Geometry: final body of the model. Coordinates: model frame, mm. Give positions to 0.01 mm unless a question says otherwise; leave off trailing zeros. Write each loop counter-clockwise with the first axis right and the second up, starting at its lowest first coordinate (ties: lowest second). Pieces come first, ordered by that corner, then holes. Notation, with made-up numbers: M -8,57.25 L 11,57.25 A28 ccw 11,93.25 Z; hole C 51,-1 d4. An arc over 180 degrees is marked long. Use a Markdown table: item, result. Add a question column.
1) Line query: line 1 (X direction, y = 36.5, z = 0.1); line 2 (Y direction, x = 25.5, z = 2.05); line 3 (Y direction, x = -25, z = 1.6). Output: solid intervals per line, ascending.
2) Pin query (flat end, axial travel): pin 1 (0.8 mm diameter, centred on x = 27.5, z = 1, fed in from +Y); pin 2 (0.8 mm diameter, centred on y = 20, z = 1.5, fed in from -X); pin 3 (1.5 mm diameter, centred on y = 12, z = 0.5, fed in from +X). Return the tip coordinate at first contact, or that it passes through.
3) Section B-B on y = 14. Return the cut outline in (x, z).
4) Section A-A on y = -15.5. Return the cut outline in (x, z), then the cut area to 3 significant figures.
```python
from build123d import *

# Parameters (mm, degrees)
F0_W        = 9.75
F0_H        = 13.75
F1_DEPTH    = 2.5
F0_W_2      = 2.5
F0_H_2      = 8
F2_DEPTH    = 1.75
F3_R        = 2
F4_R        = 5
F5_T1_DEPTH = 23.4006350946


# Not quite as in the source:
# - a fillet or chamfer that OpenCascade refuses, or shapes differently, is made with other operations: its cross-section is extruded or revolved along the edge and cut away or added


with BuildPart() as f1:
    # F0 (on Top) → F1 (new body)
    with BuildSketch(Plane.XY):
        Polygon((25.0968417823, 39.3397479696), (-25.4031582177, 39.3397479696), (-25.4031582177, 30.0897479696), (-25.4031582177, 22.0897479696), (-25.4031582177, -4.6602520304), (-25.4031582177, -12.6602520304), (-25.4031582177, -21.9102520304), (25.0968417823, -21.9102520304), (25.0968417823, 1.8397479696), (25.0968417823, 15.5897479696), align=None)
        with Locations((29.9718417823, 8.7147479696)):
            Rectangle(F0_W, F0_H)
    extrude(amount=F1_DEPTH)

    # F0 (on Top) → F2 (join)
    with BuildSketch(Plane.XY):
        with Locations((-26.6531582177, 26.0897479696)):
            Rectangle(F0_W_2, F0_H_2)
        with Locations((-26.6531582177, -8.6602520304)):
            Rectangle(F0_W_2, F0_H_2)
    extrude(amount=F2_DEPTH)

    # F3
    f3_edges = [f1.edges().sort_by_distance(p)[0] for p in [
        (-25.403158, 39.339748, 1.25),
        (-25.403158, -21.910252, 1.25),
        (25.096842, -21.910252, 1.25),
        (25.096842, 39.339748, 1.25),
    ]]
    fillet(f3_edges, radius=F3_R)

    # F4
    f4_edges = [f1.edges().sort_by_distance(p)[0] for p in [
        (34.846842, 1.839748, 1.25),
        (34.846842, 15.589748, 1.25),
    ]]
    fillet(f4_edges, radius=F4_R)

    # F5: fillet of radius 5 on 4 edges, made by hand

    # F5_s2 → F5_t1 (cut)
    with BuildSketch(Plane.XY.offset(-10.8253175473)):
        with BuildLine():
            ThreePointArc((-25.4031582177, 30.0897479696), (-27.2332852366, 28.2596209506), (-27.9031582177, 25.7596209506))
            Line((-27.9031582177, 25.7596209506), (-27.9031582177, 30.0897479696))
            Line((-27.9031582177, 30.0897479696), (-25.4031582177, 30.0897479696))
        make_face()
        with BuildLine():
            ThreePointArc((-27.9031582177, 26.4198749885), (-27.2332852366, 23.9198749885), (-25.4031582177, 22.0897479696))
            Line((-25.4031582177, 22.0897479696), (-27.9031582177, 22.0897479696))
            Line((-27.9031582177, 22.0897479696), (-27.9031582177, 26.4198749885))
        make_face()
        with BuildLine():
            ThreePointArc((-25.4031582177, -4.6602520304), (-27.2332852366, -6.4903790494), (-27.9031582177, -8.9903790494))
            Line((-27.9031582177, -8.9903790494), (-27.9031582177, -4.6602520304))
            Line((-27.9031582177, -4.6602520304), (-25.4031582177, -4.6602520304))
        make_face()
        with BuildLine():
            ThreePointArc((-25.4031582177, -12.6602520304), (-27.2332852366, -10.8301250115), (-27.9031582177, -8.3301250115))
            Line((-27.9031582177, -8.3301250115), (-27.9031582177, -12.6602520304))
            Line((-27.9031582177, -12.6602520304), (-25.4031582177, -12.6602520304))
        make_face()
    extrude(amount=F5_T1_DEPTH, mode=Mode.SUBTRACT)


solid = f1.part
```
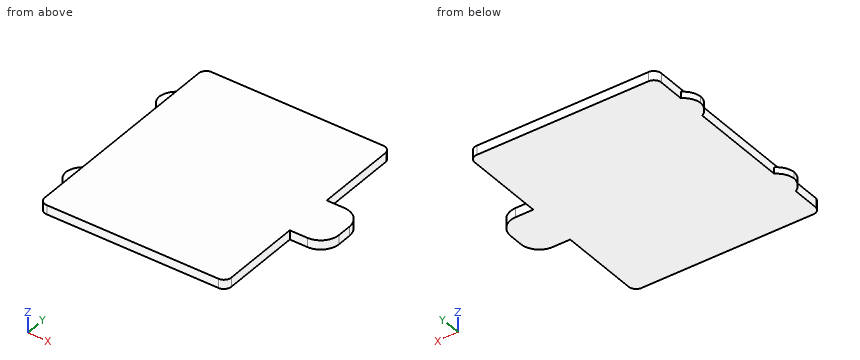
Found:
| question | item | result |
|---|---|---|
| 1 | line 1 | -25.4 to 25.1 |
| 1 | line 2 | 1.84 to 15.59 |
| 1 | line 3 | -21.11 to 38.54 |
| 2 | pin 1 | y = 15.59 |
| 2 | pin 2 | x = -25.4 |
| 2 | pin 3 | x = 34.8 |
| 3 | outline | M -25.4,0 L 33.5,0 L 33.5,2.5 L -25.4,2.5 Z |
| 4 | outline | M -25.4,0 L 25.1,0 L 25.1,2.5 L -25.4,2.5 Z |
| 4 | area | 126 mm² |
